Source: three-view drawing plus pictorial views. Frame: mm from the lowest corner of the part. Give positions to 0.01 mm unless a question says otherwise; leave off trailing zeros. Loops run counter-clockwise (first coordinate to the right, second up) from the corner with the lowest first, then second, coordinate; pieces in that order, holes last. Notation, with made-up numbers: (80, 48.25) -> (93, 48.25) arc R29 ccw to (93, 87.25) -> close; hole circle Ø10 at (84.5, -28.75). An arc over 180 degrees is marked (long way). Answer as a JSON object with one key per item and string values. Group by question number.
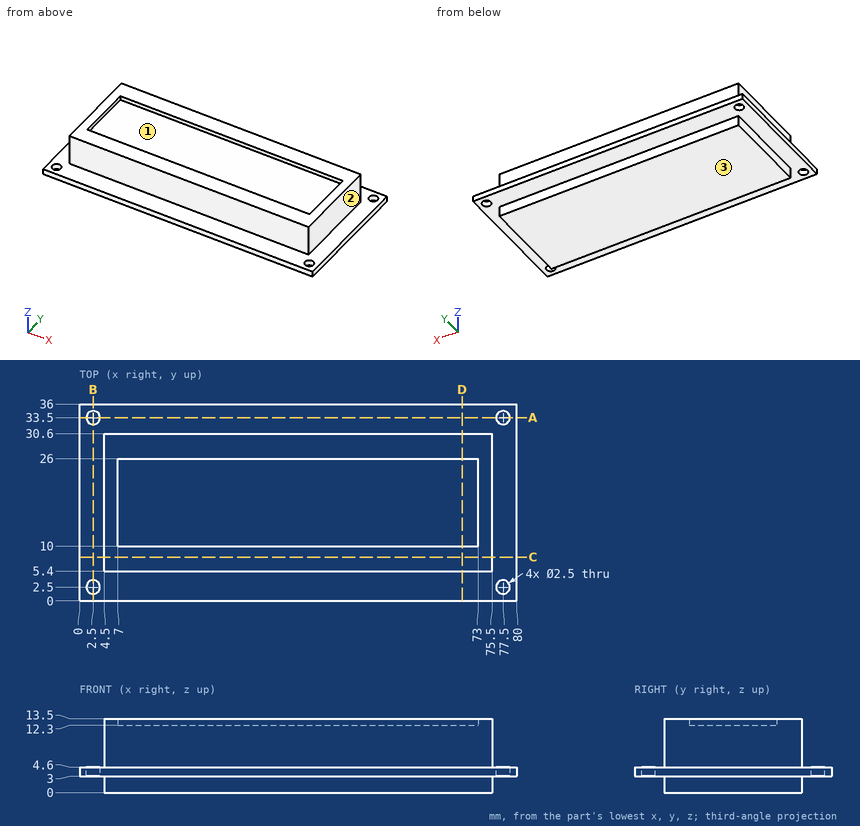
(1) Mould query, pull axis X, two halves, no side actions, for the marked faces 1, 2 and 3. Classes: pulls with the +X half, pulls with the -X half, needs draft (parallel to the pull), parting line crosses it, or undercut.
(2) Section query A-A on y = 33.5. Return the cut outline in (x, z).
(3) Section query C-C on y = 8. Return the cut outline in (x, z), plus the area to 3 significant figures.
(4) Section query D-D on x = 70. Return the cut outline in (y, z).
(5) Section query B-B on x = 2.5. Return the cut outline in (y, z), plus the area to 3 significant figures.
(6) First-contact query: pin 1 (5 mm diameter, centred on x = 37, y = 14, fed in from +Z); pin 2 (3 mm diameter, centred on y = 5, z = 10.5, fed in from -X); pin 3 (1.5 mm diameter, centred on x = 77.5, y = 33.5, fed in from -Z); pin 4 (4.5 mm diameter, centred on x = 36.5, z = 8, fed in from +Y). Flat tips, straight axial feed; report the tip coordinate or a pass-through.
(7) Material intervals for line 1 (X direction, y = 33.5, z = 3.55); line 2 (Y direction, x = 77.5, z = 3.6); line 3 (Y direction, x = 63.5, z = 2), sorted ascending. Write a range as from..to.
Result:
{
 "1": {"face 1": "undercut", "face 2": "pulls with the +X half", "face 3": "needs draft"},
 "2": {"outline": "(0, 3) -> (1.25, 3) -> (1.25, 4.6) -> (0, 4.6) -> close; (3.75, 3) -> (76.25, 3) -> (76.25, 4.6) -> (3.75, 4.6) -> close; (78.75, 3) -> (80, 3) -> (80, 4.6) -> (78.75, 4.6) -> close"},
 "3": {"outline": "(0, 3) -> (4.5, 3) -> (4.5, 0) -> (75.5, 0) -> (75.5, 3) -> (80, 3) -> (80, 4.6) -> (75.5, 4.6) -> (75.5, 13.5) -> (4.5, 13.5) -> (4.5, 4.6) -> (0, 4.6) -> close", "area": "973 mm²"},
 "4": {"outline": "(0, 3) -> (5.4, 3) -> (5.4, 0) -> (30.6, 0) -> (30.6, 3) -> (36, 3) -> (36, 4.6) -> (30.6, 4.6) -> (30.6, 13.5) -> (26, 13.5) -> (26, 12.3) -> (10, 12.3) -> (10, 13.5) -> (5.4, 13.5) -> (5.4, 4.6) -> (0, 4.6) -> close"},
 "5": {"outline": "(0, 3) -> (1.25, 3) -> (1.25, 4.6) -> (0, 4.6) -> close; (3.75, 3) -> (32.25, 3) -> (32.25, 4.6) -> (3.75, 4.6) -> close; (34.75, 3) -> (36, 3) -> (36, 4.6) -> (34.75, 4.6) -> close", "area": "49.6 mm²"},
 "6": {"pin 1": "z = 12.3", "pin 2": "x = 4.5", "pin 3": "through", "pin 4": "y = 30.6"},
 "7": {"line 1": "0..1.25, 3.75..76.25, 78.75..80", "line 2": "0..1.25, 3.75..32.25, 34.75..36", "line 3": "5.4..30.6"}
}
